```python
from build123d import *

# Parameters (mm, degrees)
SKETCH042_W   = 9
SKETCH042_H   = 28
PAD027_DEPTH  = 1
SKETCH043_W   = 9
SKETCH043_H   = 28
SKETCH043_W_2 = 7
SKETCH043_H_2 = 26
PAD028_DEPTH  = 3
BOX002_W      = 11
BOX002_H      = 30
BOX002_DEPTH  = 5


with BuildPart() as sidemold:
    # Sketch042 → Pad027 (new body)
    with BuildSketch(Plane.XY):
        Rectangle(SKETCH042_W, SKETCH042_H)
    extrude(amount=PAD027_DEPTH)

    # Sketch043 (on Face6 of Pad027) → Pad028 (join)
    with BuildSketch(Plane.XY.offset(1)):
        Rectangle(SKETCH043_W, SKETCH043_H)
        Rectangle(SKETCH043_W_2, SKETCH043_H_2, mode=Mode.SUBTRACT)
    extrude(amount=PAD028_DEPTH)


with BuildPart() as sidemold_1:
    # Body009 placement: moved
    add(sidemold.part.moved(Location((150, 35, 0))))


with BuildPart() as short_side_mold:
    # Box002 → Box002 (new body)
    with BuildSketch(Plane(origin=(144.5, 20, 0), x_dir=(1, 0, 0), z_dir=(0, 0, 1))):
        with Locations((5.5, 15)):
            Rectangle(BOX002_W, BOX002_H)
    extrude(amount=BOX002_DEPTH)

    # Cut002: cut SideMold
    add(sidemold_1.part, mode=Mode.SUBTRACT)


with BuildPart() as short_side_mold_1:
    # Cut002 placement: moved
    add(short_side_mold.part.moved(Location((0, 42, 0))))


solid = short_side_mold_1.part
```
Geometry check sheet. Reference: the model listing, model coordinates, mm. A direction names the side the tool comes from. Coordinates: 2 decimals unless noted, no trailing zeros. Write each loop counter-clockwise with the first axis right and the second up, starting at its lowest first coordinate (ties: lowest second). Pieces come first, ordered by that corner, then holes. Notation, with made-up numbers: M 16.25,3 L 27.25,3 A15 ccw 27.25,10 Z; hole C -23,60.25 d4. An arc over 180 degrees is marked long. One line per item, written item: value. Start each with the question number.
(1) Sectioned sample at B-B, the plane x = 154. Enter the section's corners in (y, z), and give its area (3 significant figures).
(2) Sectioned sample at C-C, the plane y = 65.5. Enter the section's corners in (x, z).
(3) Sectioned sample at D-D, the plane x = 148. Enter the section's corners in (y, z), and give its area (3 significant figures).
(4) Sectioned sample at A-A, the plane z = 3. Enter the section's corners in (x, y).
(5) Release check for a two-part mould opening along Y. For faces 1 (the face through (150, 62, 2)), 2 (the face through (146, 78, 4)), 3 (the face through (150, 77, 5)) record: released by +Y, released by -Y, zero draft, split by the parting line, or undercut.
(6) Scan lines: line 1 along Y through (x, z) = (151.25, 3.7); line 2 along X through (y, z) = (68, 3.8); line 3 along X through (y, z) = (78.5, 0.65). Record each from-to range of solid material in increasing order. Write a range as [from, to].
(7) Tool access check on faces 4 (the face through (145.5, 77, 2)), 5 (the face through (144.5, 77, 2)). Record the directions out of +Z, -Z, +X, -X, +Y, -Y that give a thin tool (end or side, any length) a straight path to the whole face; none if there is none.
Filled sheet:
1. outline: M 62,0 L 63,0 L 63,4 L 91,4 L 91,0 L 92,0 L 92,5 L 62,5 Z
1. area: 38.0 mm²
2. outline: M 144.5,0 L 145.5,0 L 145.5,4 L 146.5,4 L 146.5,1 L 153.5,1 L 153.5,4 L 154.5,4 L 154.5,0 L 155.5,0 L 155.5,5 L 144.5,5 Z
3. outline: M 62,0 L 63,0 L 63,4 L 64,4 L 64,1 L 90,1 L 90,4 L 91,4 L 91,0 L 92,0 L 92,5 L 62,5 Z
3. area: 116 mm²
4. outline: M 144.5,62 L 155.5,62 L 155.5,92 L 144.5,92 Z; M 146.5,64 L 153.5,64 L 153.5,90 L 146.5,90 Z; hole M 145.5,63 L 154.5,63 L 154.5,91 L 145.5,91 Z
5. face 1: released by -Y
5. face 2: undercut
5. face 3: zero draft
6. line 1: [62, 63], [64, 90], [91, 92]
6. line 2: [144.5, 145.5], [146.5, 153.5], [154.5, 155.5]
6. line 3: [144.5, 145.5], [154.5, 155.5]
7. face 4: -Z
7. face 5: +Z, -Z, -X, +Y, -Y
